from build123d import *

# Parameters (mm, degrees)
SKETCH_2_R      = 1.6
EXTRUDE_1_DEPTH = 3


with BuildPart() as part:
    # 草图2 → 凸台-拉伸1 (new body)
    with BuildSketch(Plane(origin=(0, 0, 0), x_dir=(1, 0, 0), z_dir=(0, 1, 0))):
        with BuildLine():
            Line((-94.472218138, 0), (-69.049640839, 0))
            ThreePointArc((-69.049640839, 0), (-62.504902792, 2.439153229), (-59.152888533, 8.56671922))
            ThreePointArc((-59.152888533, 8.56671922), (0, 59.77), (59.152888533, 8.56671922))
            ThreePointArc((59.152888533, 8.56671922), (62.504902792, 2.439153229), (69.049640839, 0))
            Line((69.049640839, 0), (94.472218138, 0))
            ThreePointArc((94.472218138, 0), (101.906137555, 3.311439459), (104.416662153, 11.052631579))
            ThreePointArc((104.416662153, 11.052631579), (0, 105), (-104.416662153, 11.052631579))
            ThreePointArc((-104.416662153, 11.052631579), (-101.906137555, 3.311439459), (-94.472218138, 0))
        make_face()
        with Locations(Location((0, 100, 0), (0, 0, 270))):
            Circle(SKETCH_2_R, mode=Mode.SUBTRACT)
        with Locations(Location((67.559020762, 73.727733681, 0), (0, 0, 270))):
            Circle(SKETCH_2_R, mode=Mode.SUBTRACT)
        with Locations(Location((99.619469809, 8.715574275, 0), (0, 0, 270))):
            Circle(SKETCH_2_R, mode=Mode.SUBTRACT)
        with Locations(Location((-67.559020762, 73.727733681, 0), (0, 0, 270))):
            Circle(SKETCH_2_R, mode=Mode.SUBTRACT)
        with Locations(Location((-99.619469809, 8.715574275, 0), (0, 0, 270))):
            Circle(SKETCH_2_R, mode=Mode.SUBTRACT)
        with BuildLine():
            Line((-82.613558209, 10), (-77.222101111, 10))
            ThreePointArc((-77.222101111, 10), (-71.101320206, 12.092026738), (-67.541506763, 17.492791776))
            ThreePointArc((-67.541506763, 17.492791776), (-47.72457253, 50.894185099), (-13.119593832, 68.525390606))
            ThreePointArc((-13.119593832, 68.525390606), (-7.292728703, 71.975349568), (-5, 78.347003133))
            Line((-5, 78.347003133), (-5, 83.666002653))
            ThreePointArc((-5, 83.666002653), (-8.583110521, 91.335652542), (-16.764705882, 93.509061789))
            ThreePointArc((-16.764705882, 93.509061789), (-65.125761737, 69.163828395), (-92.332800352, 22.352941176))
            ThreePointArc((-92.332800352, 22.352941176), (-90.472610689, 13.816530576), (-82.613558209, 10))
        make_face(mode=Mode.SUBTRACT)
        with BuildLine():
            Line((77.222101111, 10), (82.613558209, 10))
            ThreePointArc((82.613558209, 10), (90.472610689, 13.816530576), (92.332800352, 22.352941176))
            ThreePointArc((92.332800352, 22.352941176), (65.125761737, 69.163828395), (16.764705882, 93.509061789))
            ThreePointArc((16.764705882, 93.509061789), (8.583110521, 91.335652542), (5, 83.666002653))
            Line((5, 83.666002653), (5, 78.347003133))
            ThreePointArc((5, 78.347003133), (7.292728703, 71.975349568), (13.119593832, 68.525390606))
            ThreePointArc((13.119593832, 68.525390606), (47.72457253, 50.894185099), (67.541506763, 17.492791776))
            ThreePointArc((67.541506763, 17.492791776), (71.101320206, 12.092026738), (77.222101111, 10))
        make_face(mode=Mode.SUBTRACT)
    extrude(amount=EXTRUDE_1_DEPTH)


solid = part.part
Here's how the part is built. I have some questions about the finished solid (model axes, mm). A direction names the side the tool comes from. Round coordinates to 2 decimals unless told otherwise and drop trailing zeros. Order: outer loops, then holes, each group sorted by start corner. A loop starts at its lowest first (then second) coordinate and runs counter-clockwise, first axis right, second up. Notation, with made-up numbers: M 33,24 L 41,24 A27 cw 41,54 Z; hole C 4.25,-24 d4. An arc over 180 degrees is marked long. Return JSON: item names as keys, results as strings. Group by question number.
1. If we section it at C-C on z = -29: List the corners of the cut face in (x, y) for me, then the cut area to 3 significant figures.
2. Please list where these lines run through material, in increasing order: probe 1 along X at (y, z) = (1.45, -9); probe 2 along X at (y, z) = (1.9, -75); probe 3 along X at (y, z) = (2.2, -35).
3. If we section it at B-B on y = 2.2: State how many separate pieces and enclosed holes the cut face has, then the cut area to 3 significant figures.
4. On a 3-axis mill with a long thin cutter (end or side, diameter ignored), from which of +Z, -Z, +X, -X, +Y, -Y can I reach the whole of each face in a straight line? I mean faces 1 (the face through (-62.581, 1.479, -2.374)), 2 (the face through (0, 0, -61)), 3 (the face through (90.394, 1.479, -13.718)). Say none if no direction works.
5. If we mould it in two halves opening along X, with no side actions, what happens to faces 4 (the face through (2.154, 1.479, -104.978)), 5 (the face through (62.43, 1.479, -2.505)), 6 (the face through (-101.984, 1.479, -3.399))? For each: pulls with the +X half, pulls with the -X half, needs draft (parallel to the pull), parting line crosses it, or undercut.
6. If we section it at A-A on x = -34.5: List the corners of the cut face in (y, z) for me, then the cut area to 3 significant figures.
7. If we section it at D-D on x = 23: List the corners of the cut face in (y, z) for me, then the cut area to 3 significant figures.
8. I'm going to push flat-ended pins straight in: pin 1 Ø3.5 at (x, z) = (-99.62, -8.72) entering from -Y; pin 2 Ø0.9 at (y, z) = (1.5, -80.5) entering from +X; pin 3 Ø3 at (x, z) = (0, -100) entering from -Y. Where does each tip first touch, or does it pass through?
Reply:
{
 "1": {"outline": "M -100.92,0 L -90.47,0 L -90.47,3 L -100.92,3 Z; M -63.46,0 L -52.26,0 L -52.26,3 L -63.46,3 Z; M 52.26,0 L 63.46,0 L 63.46,3 L 52.26,3 Z; M 90.47,0 L 100.92,0 L 100.92,3 L 90.47,3 Z", "area": "130 mm^2"},
 "2": {"probe 1": "-104.42 to -101.19, -98.04 to -59.09, 59.09 to 98.04, 101.19 to 104.42", "probe 2": "-73.48 to -68.53, -66.59 to -58.31, -5.58 to 5.58, 58.31 to 66.59, 68.53 to 73.48", "probe 3": "-98.99 to -88.32, -60.36 to -48.45, 48.45 to 60.36, 88.32 to 98.99"},
 "3": {"separate pieces": "1", "enclosed holes": "7", "area": "5,990 mm^2"},
 "4": {"face 1": "+Z, +Y, -Y", "face 2": "+Z, -Z, +X, -X, -Y", "face 3": "+Y, -Y"},
 "5": {"face 4": "parting line crosses it", "face 5": "undercut", "face 6": "pulls with the -X half"},
 "6": {"outline": "M 0,-99.17 L 3,-99.17 L 3,-88.51 L 0,-88.51 Z; M 0,-60.64 L 3,-60.64 L 3,-48.81 L 0,-48.81 Z", "area": "67.5 mm^2"},
 "7": {"outline": "M 0,-102.45 L 3,-102.45 L 3,-92.17 L 0,-92.17 Z; M 0,-65.87 L 3,-65.87 L 3,-55.17 L 0,-55.17 Z", "area": "62.9 mm^2"},
 "8": {"pin 1": "y = 0", "pin 2": "x = 67.95", "pin 3": "through"}
}
